The model under review builds one solid part; all positions refer to its coordinate system, in mm. Round coordinates to 2 decimals unless told otherwise and drop trailing zeros. Write each loop counter-clockwise with the first axis right and the second up, starting at its lowest first coordinate (ties: lowest second). Pieces come first, ordered by that corner, then holes. Notation, with made-up numbers: (54, 85) -> (67, 85) arc R19 ccw to (67, 116) -> close; hole circle Ø6 at (-28.5, 47.5). An arc over 180 degrees is marked (long way). Use CSV: the item, a comma, the result in double quotes. Start each with the question number.
1) Take a section at B-B, the plane x = 42.5. Give the boundary of the cut face in (y, z), then the cut area to 3 significant figures.
2) Take a section at A-A, the plane z = -75. Give the boundary of the cut face in (x, y), then the cut area to 3 significant figures.
3) Take a section at C-C, the plane x = 123. Give the boundary of the cut face in (y, z), then the cut area to 3 significant figures.
4) For pin 1 Ø2.5 at (x, z) = (10, -10) entering from +Y; pin 2 Ø3 at (x, z) = (54.5, -15) entering from -Y, all flat-tipped, find the tip position at first contact; note any pin that passes through.
5) Wall thickness on probe 1 along X at (y, z) = (3.1, -10); probe 2 along Z at (x, y) = (100, 2.1); probe 3 along Z at (x, y) = (141, 2.7): over which ranges is each line inside the solid? List them lowest first. Write a range as [from, to].
from build123d import *

# Parameters (mm, degrees)
SKETCH1_W           = 200
SKETCH1_H           = 120
BOSS_EXTRUDE1_DEPTH = 5
SKETCH2_R           = 1
CUT_EXTRUDE1_DEPTH  = 10
SKETCH3_W           = 27
SKETCH3_H           = 40
BOSS_EXTRUDE2_DEPTH = 0.1
SKETCH4_W           = 100
SKETCH4_H           = 28
BOSS_EXTRUDE3_DEPTH = 0.1
SKETCH5_R           = 1.5
SKETCH5_W           = 5
SKETCH5_H           = 8
SKETCH5_W_2         = 10
SKETCH5_H_2         = 10
CUT_EXTRUDE2_DEPTH  = 234.293827608
SKETCH6_W           = 124
SKETCH6_H           = 39
BOSS_EXTRUDE4_DEPTH = 0.1


with BuildPart() as part:
    # Sketch1 → Boss-Extrude1 (new body)
    with BuildSketch(Plane(origin=(0, 0, 0), x_dir=(1, 0, 0), z_dir=(0, 1, 0))):
        with Locations((100, 60)):
            Rectangle(SKETCH1_W, SKETCH1_H)
    extrude(amount=BOSS_EXTRUDE1_DEPTH)

    # Sketch2 → Cut-Extrude1 (cut)
    with BuildSketch(Plane(origin=(0, 5, 0), x_dir=(1, 0, 0), z_dir=(0, 1, 0))):
        with Locations(Location((10, 110, 0), (0, 0, 270))):
            Circle(SKETCH2_R)
        with Locations(Location((190, 110, 0), (0, 0, 90))):
            Circle(SKETCH2_R)
        with Locations(Location((190, 10, 0), (0, 0, 270))):
            Circle(SKETCH2_R)
        with Locations(Location((10, 10, 0), (0, 0, 90))):
            Circle(SKETCH2_R)
    extrude(amount=-CUT_EXTRUDE1_DEPTH, mode=Mode.SUBTRACT)

    # Sketch3 → Boss-Extrude2 (add)
    with BuildSketch(Plane.XZ):
        with Locations((13.5, -60)):
            Rectangle(SKETCH3_W, SKETCH3_H)
        with Locations((186.5, -60)):
            Rectangle(SKETCH3_W, SKETCH3_H)
    extrude(amount=BOSS_EXTRUDE2_DEPTH)

    # Sketch4 → Boss-Extrude3 (add)
    with BuildSketch(Plane.XZ):
        with Locations((100, -106)):
            Rectangle(SKETCH4_W, SKETCH4_H)
    extrude(amount=BOSS_EXTRUDE3_DEPTH)

    # Sketch5 → Cut-Extrude2 (cut, through all)
    with BuildSketch(Plane.XZ.offset(0.1)):
        with Locations(Location((53, -95, 0), (0, 0, 270))):
            Circle(SKETCH5_R)
        with Locations(Location((90, -95, 0), (0, 0, 270))):
            Circle(SKETCH5_R)
        with Locations(Location((100, -95, 0), (0, 0, 270))):
            Circle(SKETCH5_R)
        with Locations(Location((110, -95, 0), (0, 0, 270))):
            Circle(SKETCH5_R)
        with Locations(Location((147, -95, 0), (0, 0, 270))):
            Circle(SKETCH5_R)
        with Locations((142.5, -102)):
            Rectangle(SKETCH5_W, SKETCH5_H)
        with Locations((68, -105)):
            Rectangle(SKETCH5_W_2, SKETCH5_H_2)
    extrude(amount=-CUT_EXTRUDE2_DEPTH, mode=Mode.SUBTRACT)

    # Sketch6 → Boss-Extrude4 (add)
    with BuildSketch(Plane(origin=(0, 5, 0), x_dir=(1, 0, 0), z_dir=(0, 1, 0))):
        with Locations((100, 24.5)):
            Rectangle(SKETCH6_W, SKETCH6_H)
    extrude(amount=BOSS_EXTRUDE4_DEPTH)


solid = part.part
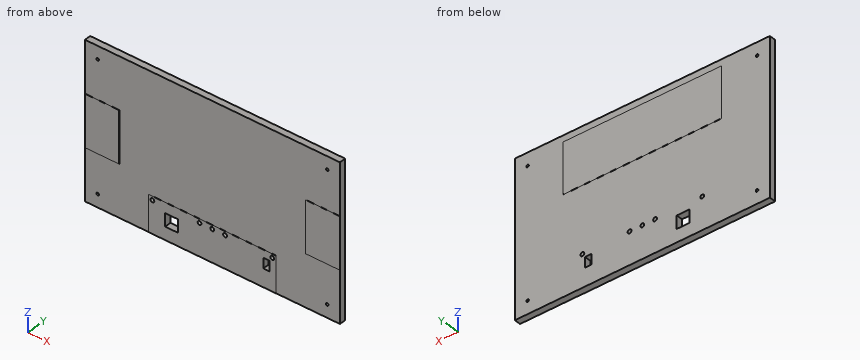
Values found:
1,outline,"(0, -120) -> (5, -120) -> (5, -44) -> (5.1, -44) -> (5.1, -5) -> (5, -5) -> (5, 0) -> (0, 0) -> close"
1,area,"604 mm²"
2,outline,"(0, -0.1) -> (27, -0.1) -> (27, 0) -> (173, 0) -> (173, -0.1) -> (200, -0.1) -> (200, 5) -> (0, 5) -> close"
2,area,"1,010 mm²"
3,outline,"(-0.1, -120) -> (5, -120) -> (5, -44) -> (5.1, -44) -> (5.1, -5) -> (5, -5) -> (5, 0) -> (0, 0) -> (0, -92) -> (-0.1, -92) -> close"
3,area,"607 mm²"
4,pin 1,"y = 5"
4,pin 2,"y = 0"
5,probe 1,"[0, 9], [11, 189], [191, 200]"
5,probe 2,"[-120, -96.5], [-93.5, 0]"
5,probe 3,"[-120, -106], [-98, 0]"
